Autodesk Inventor part; units mm, degrees
ref_plane "YZ Plane" through (0, 0, 0) normal (1, 0, 0) x (0, 1, 0)
ref_plane "XZ Plane" through (0, 0, 0) normal (0, 1, 0) x (-1, 0, 0)
ref_plane "XY Plane" through (0, 0, 0) normal (0, 0, 1) x (1, 0, 0)
sketch "スケッチ1" plane through (0, 0, 0) normal (0, 0, 1) x (1, 0, 0)
  circle A0 centre (0, 0) radius 4
  dimension "d13" = 8
extrude "押し出し1" add sketch "スケッチ1" along normal mid plane 3
sketch "スケッチ2" plane through (0, 0, 1.5) normal (0, 0, 1) x (1, 0, 0)
  point P0 (0, 0)
  point P1 (0, 0)
hole "穴1" at (0, 0, 1.5) direction (0, 0, -1) diameter 4.5 end through all
mirror "ミラー1" about plane through (0, 0, 0) normal (0, 0, 1) of "穴1"
chamfer "面取り1" distance 0.2 angle 45 4 edges at (0, 2.25, 1.5) (-4, 0, 1.5) (-4, 0, -1.5) (0, 2.25, -1.5)
properties part number "unir-spacer6" material "鋼、炭素鋼"
Model file for the job. Use its own axes, mm. Round coordinates to 2 decimals unless told otherwise and drop trailing zeros. Write each loop counter-clockwise with the first axis right and the second up, starting at its lowest first coordinate (ties: lowest second). Pieces come first, ordered by that corner, then holes. Notation, with made-up numbers: (14, -35.5) -> (26, -35.5) arc R8 ccw to (26, -22.5) -> close; hole circle Ø2 at (37.5, 42.25). An arc over 180 degrees is marked (long way). Answer as CSV lines item,"result".
1. Pin check, flat tip, straight feed: pin 1 Ø1 at (y, z) = (-2, -1) entering from +X. Stop position of the tip, or through.
Resolved:
pin 1,"x = 3.71"
2. Mould opens along X. For faces 1 (the face through (2.5, -0.8, 1.5)), 2 (the face through (-0.867, -3.905, 0.018)), 3 (the face through (-2.23, 0.29, -0.02)) say: +X half, -X half, draft (parallel to the pull), parting line (faces both ways), or undercut.
Resolved:
face 1,"draft"
face 2,"parting line"
face 3,"undercut"
3. Slice it at C-C, the plane z = -1. List the corners of the cut face in (x, y).
Resolved:
outline,"circle Ø8 at (0, 0); hole circle Ø4.5 at (0, 0)"
4. Drill centre lines: line 1 (Y direction, x = 0, z = 0.75); line 2 (X direction, y = -2, z = 0.9); line 3 (Y direction, x = -0.75, z = -0.5). Where is each one in solid material? Low to high.
Resolved:
line 1,"-4 to -2.25, 2.25 to 4"
line 2,"-3.46 to -1.03, 1.03 to 3.46"
line 3,"-3.93 to -2.12, 2.12 to 3.93"
5. Slice it at A-A, the plane y = 0. List the corners of the cut face in (x, z).
Resolved:
outline,"(-4, -1.3) -> (-3.8, -1.5) -> (-2.45, -1.5) -> (-2.25, -1.3) -> (-2.25, 1.3) -> (-2.45, 1.5) -> (-3.8, 1.5) -> (-4, 1.3) -> close; (2.25, -1.3) -> (2.45, -1.5) -> (3.8, -1.5) -> (4, -1.3) -> (4, 1.3) -> (3.8, 1.5) -> (2.45, 1.5) -> (2.25, 1.3) -> close"
